from build123d import *

# Parameters (mm, degrees)
SKETCH1_R                  = 3.429
BOSS_EXTRUDE1_DEPTH        = 12.7
F_10_24_TAPPED_HOLE1_D     = 3.7973
F_10_24_TAPPED_HOLE1_DEPTH = 19.05
F_10_24_TAPPED_HOLE1_TIP   = 1.140824014


with BuildPart() as part:
    # Sketch1 → Boss-Extrude1 (new body)
    with BuildSketch(Plane.XY):
        with BuildLine():
            Line((-38.1, -17.145), (38.1, -17.145))
            Line((38.1, -17.145), (38.1, 17.145))
            Line((38.1, 17.145), (22.561451151, 17.145))
            ThreePointArc((22.561451151, 17.145), (17.4625, 14.5796), (12.363548849, 17.145))
            Line((12.363548849, 17.145), (-12.363548849, 17.145))
            ThreePointArc((-12.363548849, 17.145), (-17.4625, 14.5796), (-22.561451151, 17.145))
            Line((-22.561451151, 17.145), (-38.1, 17.145))
            Line((-38.1, 17.145), (-38.1, -17.145))
        make_face()
        with Locations((-17.4625, -10.795)):
            Circle(SKETCH1_R, mode=Mode.SUBTRACT)
        with Locations(Location((17.4625, -10.795, 0), (0, 0, 180))):
            Circle(SKETCH1_R, mode=Mode.SUBTRACT)
        with Locations((-17.4625, 1.905)):
            Circle(SKETCH1_R, mode=Mode.SUBTRACT)
    extrude(amount=BOSS_EXTRUDE1_DEPTH)

    # #10-24 Tapped Hole1
    with Locations(Plane(origin=(0, 17.145, 0), x_dir=(1, 0, 0), z_dir=(0, 1, 0))):
        with Locations((30.48, -6.35), (-30.48, -6.35), (0, -6.35)):
            Hole(F_10_24_TAPPED_HOLE1_D / 2, depth=F_10_24_TAPPED_HOLE1_DEPTH)
            with Locations((0, 0, -(F_10_24_TAPPED_HOLE1_DEPTH + F_10_24_TAPPED_HOLE1_TIP / 2))):  # 118° drill point
                Cone(0, F_10_24_TAPPED_HOLE1_D / 2, F_10_24_TAPPED_HOLE1_TIP, mode=Mode.SUBTRACT)


solid = part.part
The listing builds one solid part. Answer for the finished solid, in the listing's coordinates (mm). A direction names the side the tool comes from. Round coordinates to 2 decimals unless told otherwise and drop trailing zeros. Write each loop counter-clockwise with the first axis right and the second up, starting at its lowest first coordinate (ties: lowest second). Pieces come first, ordered by that corner, then holes. Notation, with made-up numbers: (88, 84) - (114, 84) arc R26 cw to (114, 110) - close; hole circle Ø3 at (48, 1). An arc over 180 degrees is marked (long way). Use a Markdown table: item, result. Add a question column.
1. The part is cut by section D-D (z = 1.25). Give the number of separate pieces and of enclosed holes in the cut face, and give its area (3 significant figures).
2. The part is cut by section A-A (y = 13). Write down the section's boundary in (x, z), and give its area (3 significant figures).
3. For a pull along Z with two mould halves and no side action, classify faces 3 (the face through (-3, 17.145, 6)), 4 (the face through (-30.18, -2.85, 6.48)), 5 (the face through (-1, 0, 12.7)) as +Z half, -Z half, draft (parallel to the pull), parting line (faces both ways), or undercut.
4. Consider line 1 (Y direction, x = -17.5, z = 1.75) (3 decimals); line 2 (Z direction, x = 0, y = 13); line 3 (X direction, y = -12, z = 11). Determine where each line is inside the solid, lowest interval first.
5. Flat-ended cylindrical pins translate along their axes: P1, Ø5.5, axis at x = -17.46, y = -10.8, coming from the -Z side; P2, Ø3.5, axis at x = -30.48, z = 6.35, coming from the +Y side. Find the tip coordinate at first contact, or state that the pin passes through.
6. The part is cut by section B-B (y = 1). Write down the section's boundary in (x, z).
7. The part is cut by section C-C (x = -18.5). Write down the section's boundary in (y, z) (3 decimals), and give its area (3 significant figures).
8. A tool of negligible diameter and unlimited length cuts with its end or side. For faces 1 (the face through (-14.19, -9.77, 6.26)), 2 (the face through (28.67, 7.49, 5.78)), from which of +Z, -Z, +X, -X, +Y, -Y can it reach the whole face along a straight path? Write none if from no direction.
Reported:
| question | item | result |
|---|---|---|
| 1 | separate pieces | 1 |
| 1 | enclosed holes | 3 |
| 1 | area | 2,470 mm^2 |
| 2 | outline | (-38.1, 0) - (38.1, 0) - (38.1, 12.7) - (-38.1, 12.7) - close; hole circle Ø3.8 at (-30.48, 6.35); hole circle Ø3.8 at (0, 6.35); hole circle Ø3.8 at (30.48, 6.35) |
| 2 | area | 934 mm^2 |
| 3 | face 3 | draft |
| 3 | face 4 | undercut |
| 3 | face 5 | +Z half |
| 4 | line 1 | -17.145 to -14.224, -7.366 to -1.524, 5.334 to 14.58 |
| 4 | line 2 | 0 to 4.45, 8.25 to 12.7 |
| 4 | line 3 | -38.1 to -20.67, -14.25 to 14.25, 20.67 to 38.1 |
| 5 | P1 | through |
| 5 | P2 | y = -1.99 |
| 6 | outline | (-38.1, 0) - (-20.77, 0) - (-20.77, 12.7) - (-38.1, 12.7) - close; (-14.16, 0) - (38.1, 0) - (38.1, 12.7) - (-14.16, 12.7) - close; hole circle Ø3.8 at (-30.48, 6.35); hole circle Ø3.8 at (0, 6.35); hole circle Ø3.8 at (30.48, 6.35) |
| 7 | outline | (-17.145, 0) - (-14.063, 0) - (-14.063, 12.7) - (-17.145, 12.7) - close; (-7.527, 0) - (-1.363, 0) - (-1.363, 12.7) - (-7.527, 12.7) - close; (5.173, 0) - (14.665, 0) - (14.665, 12.7) - (5.173, 12.7) - close |
| 7 | area | 238 mm^2 |
| 8 | face 1 | +Z, -Z |
| 8 | face 2 | +Y |
